Work out the finished part from the listing and answer in its coordinate system (mm). Round coordinates to 2 decimals unless told otherwise and drop trailing zeros. Write each loop counter-clockwise with the first axis right and the second up, starting at its lowest first coordinate (ties: lowest second). Pieces come first, ordered by that corner, then holes. Notation, with made-up numbers: (4, 87.25) - (47, 87.25) arc R15 ccw to (47, 91.25) - close; hole circle Ø10 at (87.25, 27). An arc over 180 degrees is marked (long way). Answer as a JSON object with one key per item and string values.
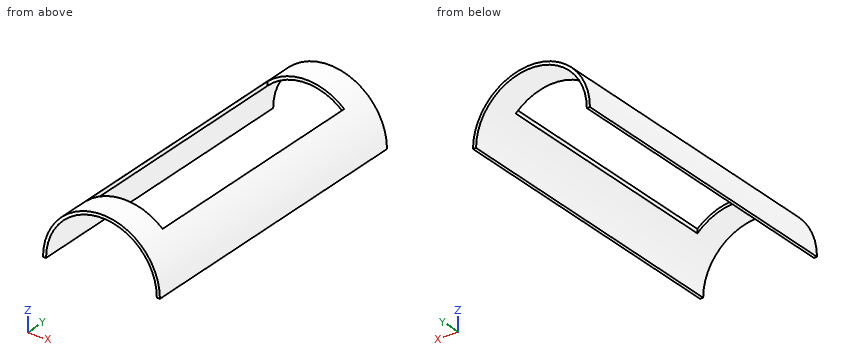
```python
from build123d import *

# Parameters (mm, degrees)
BOSS_EXTRUDE1_DEPTH     = 50
SHELL1_T                = -1
CUT_EXTRUDE1_DEPTH      = 57.762663785
CUT_EXTRUDE1_DEPTH_BACK = 57.762663785
SKETCH2_W               = 25
SKETCH2_H               = 80


with BuildPart() as part:
    # Sketch1 → Boss-Extrude1 (new, symmetric)
    with BuildSketch(Plane(origin=(0, 0, 0), x_dir=(1, 0, 0), z_dir=(0, 1, 0))):
        with BuildLine():
            Line((19, 0), (-19, 0))
            ThreePointArc((-19, 0), (0, -19), (19, 0))
        make_face()
    extrude(amount=BOSS_EXTRUDE1_DEPTH, both=True)

    # Shell1
    shell1_openings = [part.faces().sort_by_distance(p)[0] for p in [
        (0, 50, 8.06385045),
        (0, -50, 8.06385045),
        (0, 0, 0),
    ]]
    offset(amount=SHELL1_T, openings=shell1_openings)

    # Sketch2 → Cut-Extrude1 (cut, two sides: drawn at the far end of the back side and taken through both)
    with BuildSketch(Plane.XY.offset(-CUT_EXTRUDE1_DEPTH_BACK)):
        Rectangle(SKETCH2_W, SKETCH2_H)
    extrude(amount=CUT_EXTRUDE1_DEPTH + CUT_EXTRUDE1_DEPTH_BACK, mode=Mode.SUBTRACT)


solid = part.part
```
Item 1: A cutting plane is placed at B-B (x = 0). Write down the section's boundary in (y, z), and give its area (3 significant figures).
Results found:
{"outline": "(-50, 18) - (-40, 18) - (-40, 19) - (-50, 19) - close; (40, 18) - (50, 18) - (50, 19) - (40, 19) - close", "area": "20.0 mm²"}
Item 2: A cutting plane is placed at D-D (x = 16). Write down the section's boundary in (y, z), and give its area (3 significant figures).
Results found:
{"outline": "(-50, 8.25) - (50, 8.25) - (50, 10.25) - (-50, 10.25) - close", "area": "200 mm²"}
Item 3: A cutting plane is placed at A-A (y = 27). Write down the section's boundary in (x, z), and give its area (3 significant figures).
Results found:
{"outline": "(-19, 0) - (-18, 0) arc R18 cw to (-12.5, 12.95) - (-12.5, 14.31) arc R19 ccw to start; (12.5, 12.95) arc R18 cw to (18, 0) - (19, 0) arc R19 ccw to (12.5, 14.31) - close", "area": "30.7 mm²"}
Item 4: Consider line 1 along X through (y, z) = (-45, 4.75); line 2 along X through (y, z) = (-42.5, 15.25); line 3 along Z through (x, y) = (15, -13). Determine where each line is inside the solid, lowest interval first.
Results found:
{"line 1": "-18.4 to -17.36, 17.36 to 18.4", "line 2": "-11.33 to -9.56, 9.56 to 11.33", "line 3": "9.95 to 11.66"}
Item 5: A cutting plane is placed at C-C (z = 15.5). Write down the section's boundary in (x, y).
Results found:
{"outline": "(-10.99, -50) - (-9.15, -50) - (-9.15, -40) - (-10.99, -40) - close; (-10.99, 40) - (-9.15, 40) - (-9.15, 50) - (-10.99, 50) - close; (9.15, -50) - (10.99, -50) - (10.99, -40) - (9.15, -40) - close; (9.15, 40) - (10.99, 40) - (10.99, 50) - (9.15, 50) - close"}
Item 6: Each of these flat-tipped pins is pushed along its axis until it touches: P1, Ø1.8, axis at x = -5.5, z = 15.5, coming from the +Y side; P2, Ø10, axis at x = 7.5, y = 40, coming from the -Z side; P3, Ø1.1, axis at y = 5.5, z = 13.5, coming from the +X side; P4, Ø1, axis at y = 5.5, z = 7.5, coming from the -X side. Where does it stop, or does it pass through?
Results found:
{"P1": "through", "P2": "z = 12.95", "P3": "x = 13.9", "P4": "x = -17.66"}
